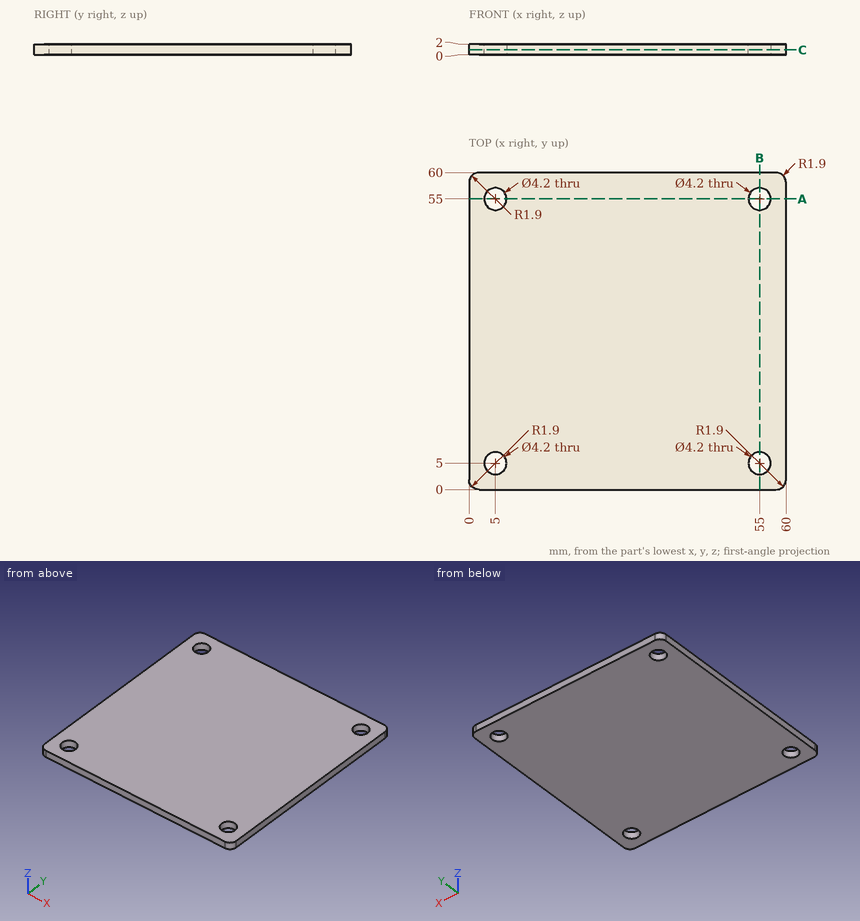
Here's the drawing with two shaded views (mm, measured from the low corner). I have some questions. Round coordinates to 2 decimals unless told otherwise and drop trailing zeros. Write each loop counter-clockwise with the first axis right and the second up, starting at its lowest first coordinate (ties: lowest second). Pieces come first, ordered by that corner, then holes.
(1) If I drill on probe 1 along Y at (x, z) = (5, 1.3); probe 2 along X at (y, z) = (6.5, 1.4), over which ranges is the centre line in solid material (lowest first)?
Findings below:
probe 1: y = 0 to 2.9, 7.1 to 52.9, 57.1 to 60
probe 2: x = 0 to 3.53, 6.47 to 53.53, 56.47 to 60
(2) Suppose I cut it at C-C on z = 0.9. Write out the boundary of the cut face in (x, y), and give its area (3 significant figures).
Findings below:
outline: (0, 1.9) arc R1.9 ccw to (1.9, 0) - (58.1, 0) arc R1.9 ccw to (60, 1.9) - (60, 58.1) arc R1.9 ccw to (58.1, 60) - (1.9, 60) arc R1.9 ccw to (0, 58.1) - close; hole circle Ø4.2 at (5, 5); hole circle Ø4.2 at (5, 55); hole circle Ø4.2 at (55, 5); hole circle Ø4.2 at (55, 55)
area: 3,540 mm2
(3) Suppose I cut it at A-A on y = 55. Write out the boundary of the cut face in (x, z).
Findings below:
outline: (0, 0) - (2.9, 0) - (2.9, 2) - (0, 2) - close; (7.1, 0) - (52.9, 0) - (52.9, 2) - (7.1, 2) - close; (57.1, 0) - (60, 0) - (60, 2) - (57.1, 2) - close
